Autodesk Inventor part; units mm, degrees
ref_plane "YZ Plane" through (0, 0, 0) normal (1, 0, 0) x (0, 1, 0)
ref_plane "XZ Plane" through (0, 0, 0) normal (0, 1, 0) x (-1, 0, 0)
ref_plane "XY Plane" through (0, 0, 0) normal (0, 0, 1) x (1, 0, 0)
sketch "Sketch1" plane through (0, 0, 0) normal (0, 1, 0) x (-1, 0, 0)
  circle A0 centre (0, 0) radius 1.75 construction
  circle A1 centre (10, 11.472032) radius 12
  line L0 (0, 0) -> (10, 11.472032) construction
  line L1 (0, 0) -> (4, 0) construction
  circle A2 centre (0, 0) radius 4 construction
  circle A3 centre (0, -11.440846) radius 6.5
  line L2 (10, 11.472032) -> (0, -11.440846) construction
  line L3 (0, 0) -> (0, -11.440846) construction
  line L4 (0, 0) -> (0, -4) construction
  line L5 (22, 11.472032) -> (22, -8.527968)
  line L6 (22, -8.527968) -> (2.703128, -17.352115)
  line L7 (-2, 11.472032) -> (-2, 6.472032)
  line L8 (-2, 6.472032) -> (-6.285281, -9.783969)
  circle A4 centre (10, 11.472032) radius 9.55
  line L9 (10, 11.472032) -> (17.5, 11.472032) construction
  circle A5 centre (17.5, 11.472032) radius 1.1
  circle A6 centre (6.25, 17.967223) radius 1.1
  circle A7 centre (6.25, 4.976842) radius 1.1
  circle A8 centre (10, 11.472032) radius 6.1
  circle A9 centre (0, -11.440846) radius 4.025
  circle A10 centre (10, 11.472032) radius 10
  circle A11 centre (0, -11.440846) radius 5
  circle A12 centre (11.624641, -6.20346) radius 7.75
  circle A13 centre (11.624641, -6.20346) radius 4.025
  circle A14 centre (19, -5.527968) radius 1.6
  circle A15 centre (19.5, 0.472032) radius 1.35
  circle A16 centre (0, -11.440846) radius 5.5
  circle A17 centre (10, 11.472032) radius 10.5
  dimension "d5" = 8
  dimension "d0" = 3.5
  dimension "d1" = 24
  dimension "d2" = 4
  dimension "d4" = 10
  dimension "d6" = 13
  dimension "d7" = 25
  dimension "d8" = 17.5
  dimension "d12" = 0
  dimension "d13" = 20
  dimension "d14" = 5
  dimension "d17" = 19.1
  dimension "d19" = 7.5
  dimension "d20" = 2.2
  dimension "d23" = 360
  dimension "d25" = 12.2
  dimension "d26" = 8.05
  dimension "d38" = 20
  dimension "d39" = 10
  dimension "d40" = 15.5
  dimension "d41" = 8.05
  dimension "d42" = 3.2
  dimension "d43" = 3
  dimension "d44" = 3
  dimension "d53" = 2.5
  dimension "d54" = 9
  dimension "d56" = 2.7
  dimension "d67" = 11
  dimension "d69" = 21
sketch "Sketch1 outline for Extrusion1" plane through (0, 0, 0) normal (0, 1, 0) x (-1, 0, 0)
  circle A0 centre (10, 11.472032) radius 6.1
  line L0 (-2, 11.472032) -> (-2, 6.472032)
  line L1 (-2, 6.472032) -> (-6.285281, -9.783969)
  arc A1 (-6.285281, -9.783969) -> (2.703128, -17.352115) centre (0, -11.440846) ccw
  line L2 (2.703128, -17.352115) -> (22, -8.527968)
  line L3 (22, -8.527968) -> (22, 11.472032)
  arc A2 (22, 11.472032) -> (-2, 11.472032) centre (10, 11.472032) ccw
extrude "Extrusion1" add sketch "Sketch1 outline for Extrusion1" against normal blind 2.5
sketch "Sketch1 outline for Extrusion2" plane through (0, 0, 0) normal (0, 1, 0) x (-1, 0, 0)
  circle A0 centre (0, -11.440846) radius 4.025
  circle A1 centre (11.624641, -6.20346) radius 4.025
extrude "Extrusion2" cut sketch "Sketch1 outline for Extrusion2" against normal blind 2.5
hole "Hole1" at (-17.5, 0, 11.472032) at (-6.25, 0, 17.967223) at (-6.25, 0, 4.976842) direction (0, -1, 0) diameter 2.2 end through all countersink diameter 4.2 countersink angle 90
hole "Hole2" at (-19, 0, -5.527968) direction (0, -1, 0) diameter 3.2 end through all countersink diameter 6.2 countersink angle 90
fillet "Fillet1" radius 5 2 edges at (-22, -1.25, -8.528) (2, -1.25, 6.472)
sketch "Sketch3" plane through (0, -2.5, 0) normal (0, -1, 0) x (1, 0, 0)
  point P0 (0, 0)
  point P1 (-19.5, 0.472032)
hole "Hole3" at (-19.5, -2.5, 0.472032) direction (0, 1, 0) diameter 2.2 end through all countersink diameter 4.2 countersink angle 90
sketch "Sketch4" plane through (0, 0, 0) normal (0, 1, 0) x (1, 0, 0)
  circle A0 centre (0, 0) radius 1.75 construction
  circle A1 centre (0, 0) radius 4 construction
  line L0 (2, -1.472032) -> (3.318061, -1.472032) construction
  line L1 (6.285281, 9.783969) -> (2.165168, -5.845474)
  arc A2 (0.568061, 0.897337) -> (0, 0) centre (3.318061, -1.472032) ccw construction
  arc A3 (-0.757721, 2.039616) -> (-1.599646, 0.709671) centre (3.318061, -1.472032) ccw
  arc A4 (1.893843, -0.244942) -> (1.599646, -0.709671) centre (3.318061, -1.472032) ccw
  arc A5 (1.893843, -0.244942) -> (-0.757721, 2.039616) centre (0.568061, 0.897337) ccw
  arc A6 (-1.599646, 0.709671) -> (1.599646, -0.709671) centre (0, 0) ccw
  line L2 (2, -1.472032) -> (2, -6.472032) construction
  dimension "d74" = 2.75
  dimension "d80" = 5
extrude "Extrusion3" cut sketch "Sketch4" against normal blind 2.5
properties part number "Dribbler Bracket"
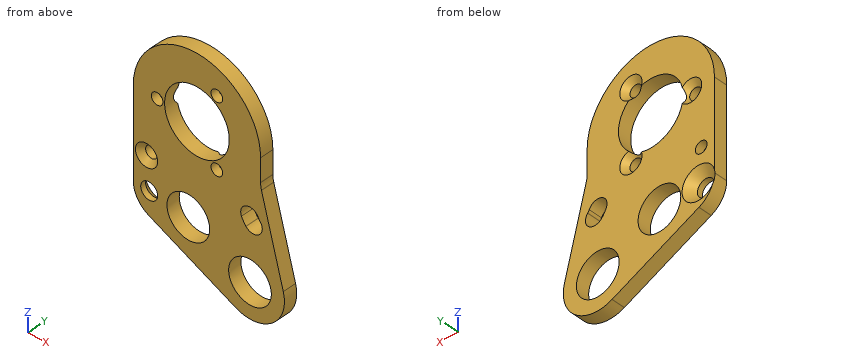
Geometry: final body of the model. Coordinates: model frame, mm. Round coordinates to 2 decimals unless told otherwise and drop trailing zeros. Loops run counter-clockwise (first coordinate to the right, second up) from the corner with the lowest first, then second, coordinate; pieces in that order, holes last.
Q1. Section C-C on x = -10. Return loops of the section in (y, z), plus the area to 3 significant figures.
Q2. Pin query (flat end, axial travel): P1, Ø1.5, axis at x = -3.5, z = -6.5, coming from the +Y side; P2, Ø2.5, axis at x = -6.25, z = 4.98, coming from the +Y side; P3, Ø1, axis at x = -2.5, y = -1.5, coming from the -Z side; P4, Ø4, axis at x = -19, z = -5.53, coming from the +Y side. Return the tip coordinate at first contact, or that it passes through.
Q3. Section A-A on z = 8. Return loops of the section in (x, y).
Q4. Section D-D on z = -15. Return loops of the section in (x, y).
Q5. Material intervals for L1, parallel to X at y = -1.3, z = -4; L2, parallel to Z at x = -19, y = -2.15; L3, parallel to Z at x = -19, y = -1.85, sorted ascending.
Q6. Section B-B on x = -6.25. Return loops of the section in (y, z), plus the area to 3 significant figures.
Evaluation:
1. outline: (-2.5, -14.02) - (0, -14.02) - (0, -9.89) - (-2.5, -9.89) - close; (-2.5, -2.52) - (0, -2.52) - (0, 5.37) - (-2.5, 5.37) - close; (-2.5, 17.57) - (0, 17.57) - (0, 23.47) - (-2.5, 23.47) - close
1. area: 44.8 mm2
2. P1: stops at y = 0
2. P2: stops at y = -0.85
2. P3: stops at z = -17.63
2. P4: stops at y = -1.1
3. outline: (-22, -2.5) - (-15.02, -2.5) - (-15.02, 0) - (-22, 0) - close; (-4.98, -2.5) - (2, -2.5) - (2, 0) - (-4.98, 0) - close
4. outline: (-7.85, -2.5) - (-1.88, -2.5) - (-1.88, 0) - (-7.85, 0) - close; (1.88, -2.5) - (5.44, -2.5) - (5.44, 0) - (1.88, 0) - close
5. L1: x = -22 to -19.95, -18.05 to -14.99, -8.26 to 4.76
5. L2: z = -9.9 to -7.13, -3.93 to -1.21, 2.15 to 19.41
5. L3: z = -9.9 to -7.13, -3.93 to -0.89, 1.83 to 19.41
6. outline: (-2.5, -15.73) - (0, -15.73) - (0, 2.88) - (-1, 3.88) - (-2.5, 3.88) - close; (-2.5, 6.08) - (-1, 6.08) - (-0.42, 6.66) - (-2.5, 6.66) - close; (-2.5, 16.28) - (-0.42, 16.28) - (-1, 16.87) - (-2.5, 16.87) - close; (-2.5, 19.07) - (-1, 19.07) - (0, 20.07) - (0, 22.87) - (-2.5, 22.87) - close
6. area: 59.6 mm2
